Autodesk Fusion 360 part; units mm, degrees
sketch "Sketch2" plane through (0, 0, 0) normal (0, 0, 1) x (1, 0, 0)
  line L0 (3, -3) -> (-3, -3)
  line L1 (-3, -3) -> (-3, 3)
  line L2 (-3, 3) -> (3, 3)
  line L3 (3, 3) -> (3, -3)
  line L4 (3, -3) -> (-3, 3) construction
  line L5 (-3, -3) -> (3, 3) construction
  dimension "d1" = 6
  dimension "d2" = 6
extrude "Extrude1" add sketch "Sketch2" along normal blind 5.8
sketch "Sketch3" plane through (0, 0, 5.8) normal (0, 0, 1) x (-1, 0, 0)
  line L0 (-3, -3) -> (3, -3)
  line L1 (3, -3) -> (3, 3)
  line L2 (3, 3) -> (-3, 3)
  line L3 (-3, 3) -> (-3, -3)
  line L4 (10, 6) -> (-10, 6)
  line L5 (-10, 6) -> (-10, -6)
  line L6 (-10, -6) -> (10, -6)
  line L7 (10, -6) -> (10, 6)
  dimension "d17" = 20
  dimension "d18" = 10
  dimension "d19" = 12
  dimension "d20" = 6
extrude "Extrude2" add sketch "Sketch3" along normal blind 1 contours L0 L1 L2 L3 | L4 L5 L6 L7
fillet "Fillet1" radius 0.25 8 edges at (0, -3, 0) (3, -3, 2.9) (3, 0, 0) (3, 3, 2.9) (0, 3, 0) (-3, 0, 0) (-3, -3, 2.9) (-3, 3, 2.9)
sketch "Sketch4" plane through (0, 0, 6.8) normal (0, 0, 1) x (-1, 0, 0)
  line L0 (10, -6) -> (10, 6)
  line L1 (10, 6) -> (-10, 6)
  line L2 (-10, 6) -> (-10, -6)
  line L3 (-10, -6) -> (10, -6)
  circle A0 centre (0, 0) radius 2.55
  dimension "d10" = 5.1
extrude "Extrude3" cut sketch "Sketch4" against normal blind 6 contours A0
fillet "Fillet2" radius 1 1 edges at (2.3774, -0.9221, 0.8)
fillet "Fillet3" radius 0.5 1 edges at (2.3774, -0.9221, 6.8)
equation "d2 = d1"
equation "d18 = d17 / 2"
equation "d20 = d19 / 2"
Geometry check sheet. Reference: the model listing, model coordinates, mm. A direction names the side the tool comes from. Round coordinates to 2 decimals unless told otherwise and drop trailing zeros. Loops run counter-clockwise (first coordinate to the right, second up) from the corner with the lowest first, then second, coordinate; pieces in that order, holes last. Notation, with made-up numbers: (-32, 68) -> (-24, 68) arc R30 ccw to (-24, 92) -> close; hole circle Ø10 at (56, -10). An arc over 180 degrees is marked (long way). Use a Markdown table: item, result.
(1) Mould release check, pull along Y, two halves, no side actions. Record for faces 1 (the flat face through (-10, 0, 6)), 2 (the flat face through (0, 0, 0.8)), 3 (the flat face through (0, 6, 6)): released by +Y, released by -Y, zero draft, split by the parting line, or undercut.
Calculated:
| item | result |
|---|---|
| face 1 | zero draft |
| face 2 | undercut |
| face 3 | released by +Y |
(2) Sectioned sample at B-B (x = 0). Enter the section's corners in (y, z), then the cut area to 3 significant figures.
Calculated:
| item | result |
|---|---|
| outline | (-6, 5.8) -> (-3, 5.8) -> (-3, 0.25) arc R0.25 ccw to (-2.75, 0) -> (2.75, 0) arc R0.25 ccw to (3, 0.25) -> (3, 5.8) -> (6, 5.8) -> (6, 6.8) -> (3.05, 6.8) arc R0.5 ccw to (2.55, 6.3) -> (2.55, 1.8) arc R1 cw to (1.55, 0.8) -> (-1.55, 0.8) arc R1 cw to (-2.55, 1.8) -> (-2.55, 6.3) arc R0.5 ccw to (-3.05, 6.8) -> (-6, 6.8) -> close |
| area | 16.5 mm² |
(3) Sectioned sample at C-C (y = 0). Enter the section's corners in (x, z), then the cut area to 3 significant figures.
Calculated:
| item | result |
|---|---|
| outline | (-10, 5.8) -> (-3, 5.8) -> (-3, 0.25) arc R0.25 ccw to (-2.75, 0) -> (2.75, 0) arc R0.25 ccw to (3, 0.25) -> (3, 5.8) -> (10, 5.8) -> (10, 6.8) -> (3.05, 6.8) arc R0.5 ccw to (2.55, 6.3) -> (2.55, 1.8) arc R1 cw to (1.55, 0.8) -> (-1.55, 0.8) arc R1 cw to (-2.55, 1.8) -> (-2.55, 6.3) arc R0.5 ccw to (-3.05, 6.8) -> (-10, 6.8) -> close |
| area | 24.5 mm² |
(4) Sectioned sample at A-A (z = 2.5). Enter the section's corners in (x, y).
Calculated:
| item | result |
|---|---|
| outline | (-3, -2.75) arc R0.25 ccw to (-2.75, -3) -> (2.75, -3) arc R0.25 ccw to (3, -2.75) -> (3, 2.75) arc R0.25 ccw to (2.75, 3) -> (-2.75, 3) arc R0.25 ccw to (-3, 2.75) -> close; hole circle Ø5.1 at (0, 0) |
(5) Set-up check for faces 4 (the cylindrical face through (-1.18, 2.26, 4.08)), 5 (the flat face through (0, -3, 3)), 6 (the flat face through (0, 3, 3)), 7 (the flat face through (-3, 0, 3)), 8 (the flat face through (3, 0, 3)): record each of +Z, -Z, +X, -X, +Y, -Y from which the full face is reachable in a straight line by a thin tool's end or side.
Calculated:
| item | result |
|---|---|
| face 4 | +Z |
| face 5 | -Z, +X, -X, -Y |
| face 6 | -Z, +X, -X, +Y |
| face 7 | -Z, -X, +Y, -Y |
| face 8 | -Z, +X, +Y, -Y |
(6) Scan lines: probe 1 along X at (y, z) = (0, 3.9); probe 2 along Z at (x, y) = (6, 1). Record each from-to range of solid material in increasing order.
Calculated:
| item | result |
|---|---|
| probe 1 | -3 to -2.55, 2.55 to 3 |
| probe 2 | 5.8 to 6.8 |
(7) Go/stop test with flat-tipped pins: P1, Ø2.5, axis at x = -0.5, y = 0.5, coming from the +Z side; P2, Ø4, axis at x = 6, y = -3, coming from the -Z side; P3, Ø1.5, axis at y = 3, z = 5, coming from the +X side. Record where each tip stops, or that it passes through.
Calculated:
| item | result |
|---|---|
| P1 | z = 0.89 |
| P2 | z = 5.8 |
| P3 | x = 3 |
(8) Sectioned sample at D-D (x = 8.5). Enter the section's corners in (y, z), then the cut area to 3 significant figures.
Calculated:
| item | result |
|---|---|
| outline | (-6, 5.8) -> (6, 5.8) -> (6, 6.8) -> (-6, 6.8) -> close |
| area | 12.0 mm² |
